```python
from build123d import *

# Parameters (mm, degrees)
SKETCH1_R                = 11.1
BOSS_EXTRUDE1_DEPTH      = 31.765
BOSS_EXTRUDE1_DEPTH_BACK = 31.765
SKETCH2_W                = 12.73
SKETCH2_H                = 38.12
BOSS_EXTRUDE2_DEPTH      = 9.43
CUT_EXTRUDE1_DEPTH       = 35.98
CHAMFER1_SIZE            = 1.6
SKETCH4_R                = 1.41
CUT_EXTRUDE2_DEPTH       = 11
SKETCH5_R                = 2.445
CUT_EXTRUDE3_DEPTH       = 13.76
SKETCH6_R                = 3.9
CUT_EXTRUDE4_DEPTH       = 4.32
SKETCH7_R                = 1.34
CUT_EXTRUDE5_DEPTH       = 7.37
SKETCH8_R                = 2
CUT_EXTRUDE6_DEPTH       = 10.5
SKETCH9_R                = 1.57
BOSS_EXTRUDE3_DEPTH      = 8.3
FILLET1_R                = 0.5
SKETCH10_R               = 1.075
CUT_EXTRUDE7_DEPTH       = 6.35


with BuildPart() as part:
    # Sketch1 → Boss-Extrude1 (new body, two sides)
    with BuildSketch(Plane(origin=(0, 0, 0), x_dir=(1, 0, 0), z_dir=(0, 1, 0))) as boss_extrude1_sk:
        Polygon((-14.34, 17.58), (-14.34, -17.4), (38.84, -17.4), (38.84, -11.03), (28.68, -11.03), (28.68, -4.64), (19.03, -4.64), (19.03, 14.49), (14.34, 14.49), (6.2, 14.49), (6.2, 17.58), align=None)
        Circle(SKETCH1_R, mode=Mode.SUBTRACT)
    extrude(amount=BOSS_EXTRUDE1_DEPTH)
    extrude(boss_extrude1_sk.sketch, amount=-BOSS_EXTRUDE1_DEPTH_BACK)

    # Sketch2 → Boss-Extrude2 (add)
    with BuildSketch(Plane.ZY.offset(14.34)):
        Rectangle(SKETCH2_W, SKETCH2_H)
    extrude(amount=BOSS_EXTRUDE2_DEPTH)

    # Sketch3 → Cut-Extrude1 (cut, through all)
    with BuildSketch(Plane(origin=(0, 0, -17.58), x_dir=(-1, 0, 0), z_dir=(0, 0, -1))):
        with BuildLine():
            Line((-38.84, 6.85), (-28.68, 19.025))
            Line((-28.68, 19.025), (-16.88, 19.025))
            ThreePointArc((-16.88, 19.025), (-15.083948776, 19.768948776), (-14.34, 21.565))
            Line((-14.34, 21.565), (-14.34, 31.765))
            Line((-14.34, 31.765), (-38.84, 31.765))
            Line((-38.84, 31.765), (-38.84, 6.85))
        make_face()
        with BuildLine():
            Line((-28.68, -19.025), (-16.88, -19.025))
            ThreePointArc((-16.88, -19.025), (-15.083948776, -19.768948776), (-14.34, -21.565))
            Line((-14.34, -21.565), (-14.34, -31.765))
            Line((-14.34, -31.765), (-38.84, -31.765))
            Line((-38.84, -31.765), (-38.84, -6.85))
            Line((-38.84, -6.85), (-28.68, -19.025))
        make_face()
    extrude(amount=-CUT_EXTRUDE1_DEPTH, mode=Mode.SUBTRACT)

    # Chamfer1
    chamfer1_edges = [part.edges().sort_by_distance(p)[0] for p in [
        (-23.77, -19.06, 0),
    ]]
    chamfer(chamfer1_edges, length=CHAMFER1_SIZE)

    # Sketch4 → Cut-Extrude2 (cut)
    with BuildSketch(Plane(origin=(0, 0, -14.49), x_dir=(-1, 0, 0), z_dir=(0, 0, -1))):
        with Locations((-12.48, 0)):
            Circle(SKETCH4_R)
    extrude(amount=-CUT_EXTRUDE2_DEPTH, mode=Mode.SUBTRACT)

    # Sketch5 → Cut-Extrude3 (cut, through all)
    with BuildSketch(Plane(origin=(0, 0, 4.64), x_dir=(-1, 0, 0), z_dir=(0, 0, -1))):
        with Locations((-23.855, -9.53)):
            Circle(SKETCH5_R)
        with Locations((-23.855, 9.53)):
            Circle(SKETCH5_R)
    extrude(amount=-CUT_EXTRUDE3_DEPTH, mode=Mode.SUBTRACT)

    # Sketch6 → Cut-Extrude4 (cut)
    with BuildSketch(Plane.XY.offset(17.4)):
        with Locations((23.855, -9.53)):
            Circle(SKETCH6_R)
        with Locations((23.855, 9.53)):
            Circle(SKETCH6_R)
    extrude(amount=-CUT_EXTRUDE4_DEPTH, mode=Mode.SUBTRACT)

    # Sketch7 → Cut-Extrude5 (cut, through all)
    with BuildSketch(Plane(origin=(0, 0, 11.03), x_dir=(-1, 0, 0), z_dir=(0, 0, -1))):
        with Locations((-34.96, 6.31)):
            Circle(SKETCH7_R)
        with Locations((-34.96, -6.31)):
            Circle(SKETCH7_R)
    extrude(amount=-CUT_EXTRUDE5_DEPTH, mode=Mode.SUBTRACT)

    # Sketch8 → Cut-Extrude6 (cut)
    with BuildSketch(Plane.ZY.offset(23.77)):
        Circle(SKETCH8_R)
    extrude(amount=-CUT_EXTRUDE6_DEPTH, mode=Mode.SUBTRACT)

    # Sketch9 → Boss-Extrude3 (add)
    with BuildSketch(Plane.ZY.offset(23.77)):
        with Locations((0, -9.505)):
            Circle(SKETCH9_R)
        with Locations((0, 9.505)):
            Circle(SKETCH9_R)
    extrude(amount=BOSS_EXTRUDE3_DEPTH)

    # Fillet1
    fillet1_edges = [part.edges().sort_by_distance(p)[0] for p in [
        (-32.07, -9.505, -1.57),
        (-32.07, 9.505, -1.57),
    ]]
    fillet(fillet1_edges, radius=FILLET1_R)

    # Sketch10 → Cut-Extrude7 (cut)
    with BuildSketch(Plane(origin=(38.84, 0, 0), x_dir=(0, 0, -1), z_dir=(1, 0, 0))):
        with Locations((-14.215, 0)):
            Circle(SKETCH10_R)
    extrude(amount=-CUT_EXTRUDE7_DEPTH, mode=Mode.SUBTRACT)


solid = part.part
```
Design review of the part built by this model. Coordinates are the model's own, in mm. A direction names the side the tool comes from. Give positions to 0.01 mm unless a question says otherwise; leave off trailing zeros. Order: outer loops, then holes, each group sorted by start corner. A loop starts at its lowest first (then second) coordinate and runs counter-clockwise, first axis right, second up. Notation, with made-up numbers: (-9.75, -22.75) -> (49.25, -22.75) arc R8 ccw to (49.25, -13.75) -> close; hole circle Ø9 at (-28, -3.75). An arc over 180 degrees is marked (long way). Write item = value, one per line. Start each with the question number.
(1) For faces 4 (the face through (22, 19.025, 8)), 5 (the face through (-27.615, -7.948, -0.204)), 6 (the face through (14.34, -27, 1)), list the 3-axis set-ups (+Z, -Z, +X, -X, +Y, -Y) from which the entire face can be reached by the end or side of a thin tool; tool diameter is ignored.
(2) For pin 1 (2 mm diameter, centred on x = -18, y = 1.5, fed in from +Z) (3 decimals); pin 2 (6 mm diameter, centred on x = 23, z = -2.5, fed in from -Y); pin 3 (6 mm diameter, centred on y = 3.5, z = -5.5, fed in from +X); pin 4 (11 mm diameter, centred on y = -28, z = 9.5, fed in from +X), all flat-tipped, find the tip position at first contact; note any pin that passes through.
(3) Mouldability with a two-part tool opening along X and no side actions: class faces 1 (the face through (-0.2, 31.765, 11.3)), 2 (the face through (36.3, -6.3, 14.2)), 3 (the face through (-32.07, -9, 0)) as +X half, -X half, draft (parallel to the pull), parting line (faces both ways), or undercut.
(4) We need section B-B on z = -8.5. Write out the cut boundary in (x, y) (3 decimals), plus the area to 3 significant figures.
(5) We need section C-C on x = 0. Write out the cut boundary in (y, z) (3 decimals).
(6) We need section D-D on y = 3.5. Write out the cut boundary in (x, z) (3 decimals).
(7) To check wall thickness, follow line 1 along X through (y, z) = (22, 0); line 2 along Z through (x, y) = (0, -17); line 3 along X through (y, z) = (-15, -13.5). State the ranges of each line that lie inside material, in increasing order.
(8) We need section A-A on x = 34.96. State how many separate pieces and enclosed holes the cut face has, plus the area to 3 significant figures.
Numbers:
q1.face_4 = +Z, -Z, +X, +Y
q1.face_5 = -X
q1.face_6 = +Z, -Z, +X, -Y
q2.pin_1 = 6.365
q2.pin_2 = through
q2.pin_3 = 19.03
q2.pin_4 = 14.34
q3.face_1 = draft
q3.face_2 = undercut
q3.face_3 = -X half
q4.outline = (-14.34, -31.765) -> (-7.139, -31.765) -> (-7.139, 31.765) -> (-14.34, 31.765) -> close; (7.139, -31.765) -> (14.34, -31.765) -> (14.34, -21.565) arc R2.54 cw to (16.88, -19.025) -> (19.03, -19.025) -> (19.03, 19.025) -> (16.88, 19.025) arc R2.54 cw to (14.34, 21.565) -> (14.34, 31.765) -> (7.139, 31.765) -> close; hole circle Ø2.82 at (12.48, 0)
q4.area = 1,090 mm^2
q5.outline = (-31.765, -17.58) -> (31.765, -17.58) -> (31.765, -11.1) -> (-31.765, -11.1) -> close; (-31.765, 11.1) -> (31.765, 11.1) -> (31.765, 17.4) -> (-31.765, 17.4) -> close
q6.outline = (-23.77, -6.365) -> (-14.34, -6.365) -> (-14.34, -17.58) -> (6.2, -17.58) -> (6.2, -14.49) -> (19.03, -14.49) -> (19.03, 4.64) -> (28.68, 4.64) -> (28.68, 11.03) -> (38.84, 11.03) -> (38.84, 17.4) -> (-14.34, 17.4) -> (-14.34, 6.365) -> (-23.77, 6.365) -> close; hole circle Ø22.2 at (0, 0)
q7.line_1 = -14.34 to -11.1, 11.1 to 14.34
q7.line_2 = -17.58 to -11.1, 11.1 to 17.4
q7.line_3 = -14.34 to 19.03
q8.separate_pieces = 3
q8.enclosed_holes = 1
q8.area = 109 mm^2
